Autodesk Inventor part; units mm, degrees
ref_plane "Work Plane2" through (-2.9972, 0.3821, 0) normal (1, 0, 0) x (0, 0, 1)
ref_plane "YZ Plane" through (0, 0, 0) normal (1, 0, 0) x (0, 1, 0)
ref_plane "XZ Plane" through (0, 0, 0) normal (0, 1, 0) x (-1, 0, 0)
sketch "Sketch1" plane through (0, 0, 0) normal (0, 0, 1) x (1, 0, 0)
  line L0 (9.5028, 23.3821) -> (9.5028, -12.6179)
  line L1 (14.5028, 23.3821) -> (14.5028, -12.6179)
  line L2 (26.5028, -12.6179) -> (26.5028, -37.6179)
  line L3 (-32.4972, -17.6179) -> (26.5028, -17.6179)
  line L4 (-32.4972, -12.6179) -> (-20.4972, -12.6179)
  line L5 (-15.4972, -12.6179) -> (9.5028, -12.6179)
  line L6 (14.5028, -12.6179) -> (26.5028, -12.6179)
  line L7 (-20.4972, 23.3821) -> (14.5028, 23.3821)
  line L8 (-15.4972, 23.3821) -> (-15.4972, -12.6179)
  line L9 (-20.4972, 23.3821) -> (-20.4972, -12.6179)
  line L10 (-32.4972, -37.6179) -> (26.5028, -37.6179)
  line L11 (-32.4972, -12.6179) -> (-32.4972, -37.6179)
  line L12 (-2.9972, 1.3821) -> (-2.9972, 17.3821) construction
  line L13 (5.0028, 9.3821) -> (-10.9972, 9.3821) construction
  circle A0 centre (-2.9972, 9.3821) radius 8 construction
  line L14 (-2.9972, 10.3821) -> (-2.9972, 8.3821) construction
  line L15 (-8.4972, 10.3821) -> (-8.4972, 8.3821)
  line L16 (2.5028, 8.3821) -> (2.5028, 10.3821)
  line L17 (-2.9972, 2.3821) -> (-2.9972, 0.3821) construction
  line L18 (-4.7472, 2.3821) -> (-4.7472, 0.3821)
  line L19 (-1.2472, 0.3821) -> (-1.2472, 2.3821)
  arc A1 (-4.7472, 0.3821) -> (-1.2472, 0.3821) centre (-2.9972, 0.3821) ccw
  line L20 (-10.9972, 10.3821) -> (-10.9972, 8.3821) construction
  line L21 (-12.7472, 10.3821) -> (-12.7472, 8.3821)
  line L22 (-9.2472, 8.3821) -> (-9.2472, 10.3821)
  arc A2 (-9.2472, 10.3821) -> (-12.7472, 10.3821) centre (-10.9972, 10.3821) ccw
  arc A3 (-12.7472, 8.3821) -> (-9.2472, 8.3821) centre (-10.9972, 8.3821) ccw
  line L23 (5.0028, 10.3821) -> (5.0028, 8.3821) construction
  line L24 (3.2528, 10.3821) -> (3.2528, 8.3821)
  line L25 (6.7528, 8.3821) -> (6.7528, 10.3821)
  arc A4 (6.7528, 10.3821) -> (3.2528, 10.3821) centre (5.0028, 10.3821) ccw
  arc A5 (3.2528, 8.3821) -> (6.7528, 8.3821) centre (5.0028, 8.3821) ccw
  line L26 (-2.9972, 18.3821) -> (-2.9972, 16.3821) construction
  line L27 (-1.2472, 18.3821) -> (-1.2472, 16.3821)
  line L28 (-4.7472, 16.3821) -> (-4.7472, 18.3821)
  arc A6 (-1.2472, 18.3821) -> (-4.7472, 18.3821) centre (-2.9972, 18.3821) ccw
  arc A7 (-1.2472, 2.3821) -> (-1.4087, 3.1165) centre (-2.9972, 2.3821) ccw
  arc A8 (-4.5856, 3.1165) -> (-4.7472, 2.3821) centre (-2.9972, 2.3821) ccw
  arc A9 (-8.4972, 8.3821) -> (-4.5856, 3.1165) centre (-2.9972, 8.3821) ccw
  arc A10 (-1.4087, 3.1165) -> (2.5028, 8.3821) centre (-2.9972, 8.3821) ccw
  arc A11 (-4.7472, 16.3821) -> (-4.5856, 15.6478) centre (-2.9972, 16.3821) ccw
  arc A12 (-1.4087, 15.6478) -> (-1.2472, 16.3821) centre (-2.9972, 16.3821) ccw
  arc A13 (2.5028, 10.3821) -> (-1.4087, 15.6478) centre (-2.9972, 10.3821) ccw
  arc A14 (-4.5856, 15.6478) -> (-8.4972, 10.3821) centre (-2.9972, 10.3821) ccw
  point P0 (0, 0)
  point P1 (14.5028, 29.202)
  point P2 (-20.4972, 29.202)
  dimension "d51" = 16
  dimension "d52" = 5
  dimension "d53" = 5
  dimension "d54" = 25
  dimension "d55" = 5
  dimension "d56" = 20
  dimension "d58" = 27
  dimension "d59" = 14
  dimension "d60" = 12
  dimension "d61" = 12
  dimension "d64" = 12.5
  dimension "d66" = 2
  dimension "d67" = 3.5
  dimension "d68" = 2
  dimension "d69" = 3.5
  dimension "d70" = 2
  dimension "d71" = 3.5
  dimension "d72" = 2
  dimension "d73" = 3.5
  dimension "d74" = 2
extrude "Extrusion1" add sketch "Sketch1" along normal blind 5
sketch "Sketch2" plane through (0, 0, 5) normal (0, 0, 1) x (1, 0, 0)
  line L0 (26.5028, -37.6179) -> (26.5028, -12.6179)
  line L1 (-32.4972, -12.6179) -> (26.5028, -12.6179)
  line L2 (26.5028, -12.6179) -> (26.5028, -17.6179)
  line L3 (26.5028, -17.6179) -> (-32.4972, -17.6179)
  line L4 (-32.4972, -17.6179) -> (-32.4972, -12.6179)
  line L5 (-32.4972, -12.6179) -> (-32.4972, -37.6179)
  line L6 (26.5028, -12.6179) -> (14.5028, -12.6179)
  point P0 (0, 0)
  dimension "d30" = 5
extrude "Extrusion2" add sketch "Sketch2" along normal blind 16
sketch "Sketch3" plane through (14.5028, -12.6179, 0) normal (1, 0, 0) x (0, 0, -1)
  line L0 (0, 0) -> (-21, 0)
  line L1 (-5, 0) -> (-5, 36)
  line L2 (-21, 0) -> (-5, 0)
  line L3 (-5, 36) -> (-20, 0)
  point P0 (0, 12.6179)
  point P1 (-5, 31)
  dimension "d77" = 15
extrude "Extrusion3" add sketch "Sketch3" against normal blind 5
sketch "Sketch4" plane through (14.5028, -12.6179, 0) normal (0, 1, 0) x (1, 0, 0)
  circle A0 centre (6, -15) radius 2.6
  line L0 (12, 0) -> (12, -21)
  line L1 (12, -21) -> (-47, -21)
  point P0 (-14.5028, 0)
  point P1 (0, -25)
  dimension "d36" = 5.2
  dimension "d37" = 6
  dimension "d38" = 6
extrude "Extrusion4" cut sketch "Sketch4" against normal through all
sketch "Sketch5" plane through (0, 0, 5) normal (0, 0, 1) x (1, 0, 0)
  arc A0 (19.0028, -25.0179) -> (19.0028, -30.2179) centre (19.0028, -27.6179) ccw
  line L0 (26.5028, -37.6179) -> (26.5028, -17.6179)
  line L1 (-32.4972, -37.6179) -> (26.5028, -37.6179)
  line L2 (19.0028, -25.0179) -> (26.5028, -25.0179)
  line L3 (19.0028, -30.2179) -> (26.5028, -30.2179)
  line L4 (26.5028, -37.6179) -> (26.5028, -12.6179)
  line L5 (26.5028, -25.0179) -> (26.5028, -30.2179)
  point P0 (0, 0)
  point P1 (-34.4972, -33.6179)
  point P2 (17.5028, -33.6179)
  dimension "d41" = 7.5
  dimension "d42" = 10
  dimension "d43" = 5.2
extrude "Extrusion5" cut sketch "Sketch5" against normal blind 5
fillet "Fillet1" radius 1 5 edges at (-32.4972, -12.6179, 10.5) (-32.4972, -17.6179, 13) (26.5028, -30.2179, 2.5) (26.5028, -25.0179, 2.5) (26.5028, -17.6179, 13)
ref_plane "Work Plane2" through (-2.9972, 0.3821, 0) normal (1, 0, 0) x (0, 0, 1)
mirror "Mirror2" about plane through (-2.9972, 0.3821, 0) normal (1, 0, 0) of "Extrusion5", "Extrusion4", "Extrusion3"
fillet "Fillet2" radius 1 8 edges at (14.5028, 23.3821, 2.5) (-20.4972, 23.3821, 2.5) (26.5028, -37.6179, 2.5) (-32.4972, -37.6179, 2.5) (-1.4087, 3.1165, 2.5) (-4.5856, 3.1165, 2.5) (-1.4087, 15.6478, 2.5) (-4.5856, 15.6478, 2.5)
ref_plane "Work Plane3" through (-2.9972, -12.6179, 0) normal (-1, 0, 0) x (0, 0, 1)
properties part number "Z Nut Braket 1.0" material "PC/ABS Plastic"
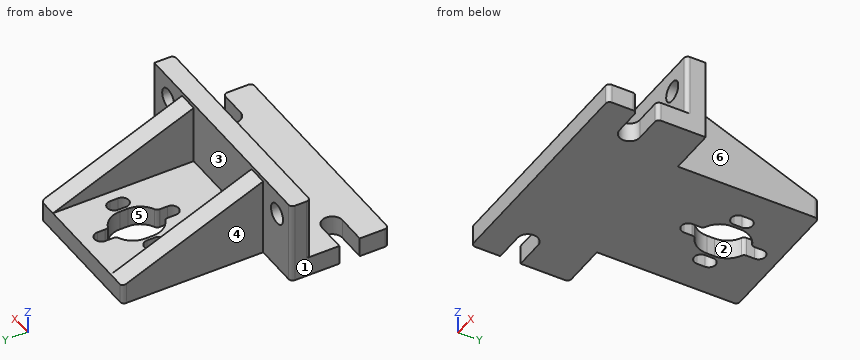
Can you work these out from the model? Positions are in its coordinate system, mm. Face numbers are marked on the shaded views. A direction names the side the tool comes from. Coordinates: 2 decimals unless noted, no trailing zeros. Write each loop counter-clockwise with the first axis right and the second up, starting at its lowest first coordinate (ties: lowest second). Pieces come first, ordered by that corner, then holes. Notation, with made-up numbers: (-13, 51.5) - (39, 51.5) arc R18 ccw to (39, 61.5) - close; hole circle Ø6 at (-18.75, 19). An arc over 180 degrees is marked (long way). Return JSON: item names as keys, results as strings. Group by question number.
Item 1: Please list where these lines run through material, in increasing order: probe 1 along X at (y, z) = (-14.6, 15); probe 2 along Y at (x, z) = (20, 2.25); probe 3 along X at (y, z) = (2.5, 6).
Item 2: Which directions (+Z, -Z, +X, -X, +Y, -Y) give clear straight access to the entire face, cutting with the end or side of a thin tool? Please do the marked faces 4, 5 and 6.
Item 3: We'd pull the mould along Y, two halves only. Please class the marked faces 1, 2 and 3: pulls with the +Y half, pulls with the -Y half, needs draft (parallel to the pull), parting line crosses it, or undercut.
Item 4: If we section it at C-C (y = 13): Write out the boundary of the cut face in (x, z), then the cut area to 3 significant figures.
Item 5: If we section it at B-B (x = -17): Write out the boundary of the cut face in (y, z).
Item 6: I'm going to push flat-ended pins straight in: pin 1 Ø4 at (y, z) = (-3.5, 4) entering from +X; pin 2 Ø4 at (x, z) = (-28, 2) entering from +Y; pin 3 Ø5 at (x, z) = (19, 9.5) entering from -Y. Where does each tip first touch, or does it pass through?
Item 7: If we section it at A-A (x = 5): Write out the boundary of the cut face in (y, z), then the cut area to 4 significant figures.
Item 8: If we section it at D-D (z = 3.5): Count the separate pieces of the cut face and the enclosed holes in it, then the cut area to 3 significant figures.
Return value:
{
 "1": {"probe 1": "x = -32.5 to -29.1, -23.9 to 17.9, 23.1 to 26.5", "probe 2": "y = -37.62 to -30.22, -25.02 to -12.62", "probe 3": "x = -20.5 to -15.5, 9.5 to 14.5"},
 "2": {"face 4": "+Z, -Z, -X, +Y", "face 5": "+Z, -Z", "face 6": "+Z, -Z, +X, +Y"},
 "3": {"face 1": "needs draft", "face 2": "undercut", "face 3": "pulls with the +Y half"},
 "4": {"outline": "(-20.5, 0) - (-7.83, 0) - (-7.83, 5) - (-15.5, 5) - (-15.5, 9.33) - (-20.5, 9.33) - close; (1.84, 0) - (14.5, 0) - (14.5, 9.33) - (9.5, 9.33) - (9.5, 5) - (1.84, 5) - close", "area": "170 mm^2"},
 "5": {"outline": "(-37.62, 0) - (23.38, 0) - (23.38, 5) - (-12.62, 20) - (-12.62, 21) - (-17.62, 21) - (-17.62, 5) - (-37.62, 5) - close"},
 "6": {"pin 1": "stops at x = 14.5", "pin 2": "stops at y = -12.62", "pin 3": "stops at y = -17.62"},
 "7": {"outline": "(-37.62, 0) - (6.63, 0) - (6.63, 5) - (-12.62, 5) - (-12.62, 21) - (-17.62, 21) - (-17.62, 5) - (-37.62, 5) - close; (12.13, 0) - (23.38, 0) - (23.38, 5) - (12.13, 5) - close", "area": "357.5 mm^2"},
 "8": {"separate pieces": "1", "enclosed holes": "3", "area": "2,460 mm^2"}
}
